Geometry check sheet. Reference: the model listing, model coordinates, mm. A direction names the side the tool comes from. Coordinates: 2 decimals unless noted, no trailing zeros. Loops run counter-clockwise (first coordinate to the right, second up) from the corner with the lowest first, then second, coordinate; pieces in that order, holes last.
from build123d import *

# Parameters (mm, degrees)
SKETCH1_R               = 24.5
BOSS_EXTRUDE1_DEPTH     = 80
FILLET1_R               = 8
CUT_EXTRUDE1_DEPTH      = 88.180846548
CUT_EXTRUDE1_DEPTH_BACK = 88.180846548
SKETCH2_R               = 5
SKETCH3_W               = 56.031714123
SKETCH3_H               = 10
CUT_EXTRUDE2_DEPTH      = 60
SKETCH4_R               = 3
CUT_EXTRUDE3_DEPTH      = 60
SKETCH5_W               = 5
SKETCH5_H               = 7
BOSS_EXTRUDE2_DEPTH     = 30
SKETCH6_R               = 2
CUT_EXTRUDE4_DEPTH      = 116.884640959


with BuildPart() as part:
    # Sketch1 → Boss-Extrude1 (new body)
    with BuildSketch(Plane(origin=(0, 0, 0), x_dir=(1, 0, 0), z_dir=(0, 1, 0))):
        with Locations(Location((0, 0, 0), (0, 0, 270))):
            Circle(SKETCH1_R)
    extrude(amount=BOSS_EXTRUDE1_DEPTH)

    # Fillet1
    fillet1_edges = [part.edges().sort_by_distance(p)[0] for p in [
        (0, 80, -24.5),
    ]]
    fillet(fillet1_edges, radius=FILLET1_R)

    # Sketch2 → Cut-Extrude1 (cut, two sides: drawn at the far end of the back side and taken through both)
    with BuildSketch(Plane.XY.offset(-CUT_EXTRUDE1_DEPTH_BACK)):
        with Locations((0, 30.57)):
            Circle(SKETCH2_R)
    extrude(amount=CUT_EXTRUDE1_DEPTH + CUT_EXTRUDE1_DEPTH_BACK, mode=Mode.SUBTRACT)

    # Sketch3 → Cut-Extrude2 (cut)
    with BuildSketch(Plane(origin=(0, 0, 0), x_dir=(1, 0, 0), z_dir=(0, 1, 0))):
        with Locations((-1.359495315, 0)):
            Rectangle(SKETCH3_W, SKETCH3_H)
    extrude(amount=CUT_EXTRUDE2_DEPTH, mode=Mode.SUBTRACT)

    # Sketch4 → Cut-Extrude3 (cut)
    with BuildSketch(Plane(origin=(0, 80, 0), x_dir=(1, 0, 0), z_dir=(0, 1, 0))):
        with Locations(Location((0, 0, 0), (0, 0, 270))):
            Circle(SKETCH4_R)
    extrude(amount=-CUT_EXTRUDE3_DEPTH, mode=Mode.SUBTRACT)

    # Sketch5 → Boss-Extrude2 (add)
    with BuildSketch(Plane(origin=(0, 80, 0), x_dir=(1, 0, 0), z_dir=(0, 1, 0))):
        with Locations((0, 8.5)):
            Rectangle(SKETCH5_W, SKETCH5_H)
    boss_extrude2 = extrude(amount=BOSS_EXTRUDE2_DEPTH)

    # Sketch6 → Cut-Extrude4 (cut, through all)
    with BuildSketch(Plane.ZY.offset(2.5)):
        with Locations((-8.5, 107)):
            Circle(SKETCH6_R)
    cut_extrude4 = extrude(amount=-CUT_EXTRUDE4_DEPTH, mode=Mode.SUBTRACT)

    # Mirror1: Boss-Extrude2, Cut-Extrude4 across plane
    add(boss_extrude2.mirror(Plane.XY))
    add(cut_extrude4.mirror(Plane.XY), mode=Mode.SUBTRACT)


solid = part.part
1) Section check C-C on y = 96. Record the cut outline in (x, z), and give its area (3 significant figures).
Data:
outline: (-2.5, -12) - (2.5, -12) - (2.5, -5) - (-2.5, -5) - close; (-2.5, 5) - (2.5, 5) - (2.5, 12) - (-2.5, 12) - close
area: 70.0 mm2
2) Section check D-D on y = 30.57. Record the cut outline in (x, z), and give its area (3 significant figures).
Data:
outline: (-23.98, -5) arc R24.5 ccw to (-5, -23.98) - (-5, -5) - close; (-23.98, 5) - (-5, 5) - (-5, 23.98) arc R24.5 ccw to start; (5, -23.98) arc R24.5 ccw to (23.98, -5) - (5, -5) - close; (5, 5) - (23.98, 5) arc R24.5 ccw to (5, 23.98) - close
area: 1,010 mm2
3) Section check A-A on x = 0. Count the separate pieces of the cut face and the enclosed holes in it, and give its area (3 significant figures).
Data:
separate pieces: 4
enclosed holes: 2
area: 3,180 mm2
4) Section check B-B on z = 0. Record the cut outline in (x, y), and give its area (3 significant figures).
Data:
outline: (-24.5, 60) - (-3, 60) - (-3, 80) - (-16.5, 80) arc R8 ccw to (-24.5, 72) - close; (3, 60) - (24.5, 60) - (24.5, 72) arc R8 ccw to (16.5, 80) - (3, 80) - close
area: 833 mm2
5) Mould release check, pull along Z, two halves, no side actions. Record for faces 1 (the flat face through (0, 0, -13)), 2 (the flat face through (0, 95, 12)), 3 (the cylindrical face through (-0.035, 108.983, -8.76)): +Z half, -Z half, draft (parallel to the pull), parting line (faces both ways), or undercut.
Data:
face 1: draft
face 2: +Z half
face 3: undercut
6) Depth check by flat-ended pin: pin 1 (7.5 mm diameter, centred on y = 98, z = 8.5, fed in from -X); pin 2 (12 mm diameter, centred on x = -7, y = 30, fed in from +Z); pin 3 (6 mm diameter, centred on x = -18.5, y = 60.5, fed in from -Z); pin 4 (5.5 mm diameter, centred on x = 0, z = 0, fed in from -Y). Enter the tip coordinate at first touch or a pass-through.
Data:
pin 1: stops at x = -2.5
pin 2: stops at z = 24.38
pin 3: stops at z = -18.97
pin 4: passes through
7) Access from +Z, -Z, +X, -X, +Y, -Y to the whole of each face (thin tool, end or side, straight path). Record for faces 4 (the flat face through (0, 95, 5)), 5 (the flat face through (-2.5, 95, -8)), 6 (the flat face through (-6, 30, -5)), 7 (the flat face through (0, 95, -12)).
Data:
face 4: +X, -X, +Y
face 5: +Z, -Z, -X, +Y
face 6: +X, -X, -Y
face 7: -Z, +X, -X, +Y
8) Material ranges on probe 1 along X at (y, z) = (66, 0); probe 2 along Y at (x, z) = (-1.25, 8.5); probe 3 along Y at (x, z) = (9.5, 9.5), recorded low to high.
Data:
probe 1: x = -24.5 to -3, 3 to 24.5
probe 2: y = 0 to 25.73, 35.41 to 105, 109 to 110
probe 3: y = 0 to 80
